Geometry check sheet. Reference: the model listing, model coordinates, mm. Coordinates: 2 decimals unless noted, no trailing zeros. Write each loop counter-clockwise with the first axis right and the second up, starting at its lowest first coordinate (ties: lowest second). Pieces come first, ordered by that corner, then holes. Notation, with made-up numbers: M 53.5,-2.75 L 70.5,-2.75 A20 cw 70.5,22.25 Z; hole C 89,-16 d10. An arc over 180 degrees is marked long. Put each result on its own line as item: value. Start each with the question number.
1) Cross-section at A-A on z = 8.5. Record the cut outline in (x, y), plus the area to 3 significant figures.
2) Scan lines: line 1 along X through (y, z) = (4.25, 2.25); line 2 along X through (y, z) = (3.5, -7.75); line 3 along Z through (x, y) = (6.5, 1). Record each from-to range of solid material in increasing order.
3) Gauge pin test, flat ends, axial feed: pin 1 (4 mm diameter, centred on y = 3, z = -3, fed in from -X); pin 2 (1.5 mm diameter, centred on y = 2.5, z = -2, fed in from +X); pin 3 (1.5 mm diameter, centred on x = -6, y = 5, fed in from +Z). Record the tip position at first contact, or that the pin passes through.
4) Cross-section at B-B on x = -4.5. Record the cut outline in (y, z).
from build123d import *

# Parameters (mm, degrees)
SKETCH_1_W               = 20
SKETCH_1_H               = 20
EXTRUDE_1_DEPTH          = 8.3
SKETCH_2_OUTSIDE_W       = 27.896
SKETCH_2_OUTSIDE_H       = 16.196
CUT_EXTRUDE_1_DEPTH      = 24.851415052
CUT_EXTRUDE_2_DEPTH      = 17.397865715
CUT_EXTRUDE_2_DEPTH_BACK = 17.397865715
SKETCH_3_OUTSIDE_W       = 27.896
SKETCH_3_OUTSIDE_H       = 16.196


with BuildPart() as part:
    # 草图1 → 凸台-拉伸1 (new body)
    with BuildSketch(Plane(origin=(0, 0, 0), x_dir=(1, 0, 0), z_dir=(0, 1, 0))):
        Rectangle(SKETCH_1_W, SKETCH_1_H)
    extrude(amount=EXTRUDE_1_DEPTH)

    # 草图2 outside → 切除-拉伸1 (cut, through all)
    with BuildSketch(Plane.XY.offset(10)):
        with Locations((0, 4.15)):
            Rectangle(SKETCH_2_OUTSIDE_W, SKETCH_2_OUTSIDE_H)
        Polygon((-10, 0), (-7, 8.3), (7, 8.3), (10, 0), align=None, mode=Mode.SUBTRACT)
    extrude(amount=-CUT_EXTRUDE_1_DEPTH, mode=Mode.SUBTRACT)

    # 草图3 outside → 切除-拉伸2 (cut, two sides: drawn at the far end of the back side and taken through both)
    with BuildSketch(Plane(origin=(0, 0, 0), x_dir=(0, 0, -1), z_dir=(1, 0, 0)).offset(-CUT_EXTRUDE_2_DEPTH_BACK)):
        with Locations((0, 4.15)):
            Rectangle(SKETCH_3_OUTSIDE_W, SKETCH_3_OUTSIDE_H)
        Polygon((-10, 0), (10, 0), (7, 8.3), (-7, 8.3), align=None, mode=Mode.SUBTRACT)
    extrude(amount=CUT_EXTRUDE_2_DEPTH + CUT_EXTRUDE_2_DEPTH_BACK, mode=Mode.SUBTRACT)


solid = part.part
Answer key:
1. outline: M -10,0 L 10,0 L 8.5,4.15 L -8.5,4.15 Z
1. area: 76.8 mm²
2. line 1: x = -8.46 to 8.46
2. line 2: x = -8.73 to 8.73
2. line 3: z = -9.64 to 9.64
3. pin 1: stops at x = -9.64
3. pin 2: stops at x = 9.37
3. pin 3: stops at z = 8.46
4. outline: M 0,-10 L 8.3,-7 L 8.3,7 L 0,10 Z
